The drawing under review shows one solid part. Ordinate dimensions are in mm from its lowest x, y, z. A direction names the side the tool comes from. Give positions to 0.01 mm unless a question says otherwise; leave off trailing zeros. Write each loop counter-clockwise with the first axis right and the second up, starting at its lowest first coordinate (ties: lowest second). Pieces come first, ordered by that corner, then holes. Notation, with made-up numbers: (53, -40) -> (59, -40) arc R19 cw to (59, -4) -> close; hole circle Ø11 at (59, 31.5). An arc over 180 degrees is marked (long way). Answer as a JSON object with one key per item and string values.
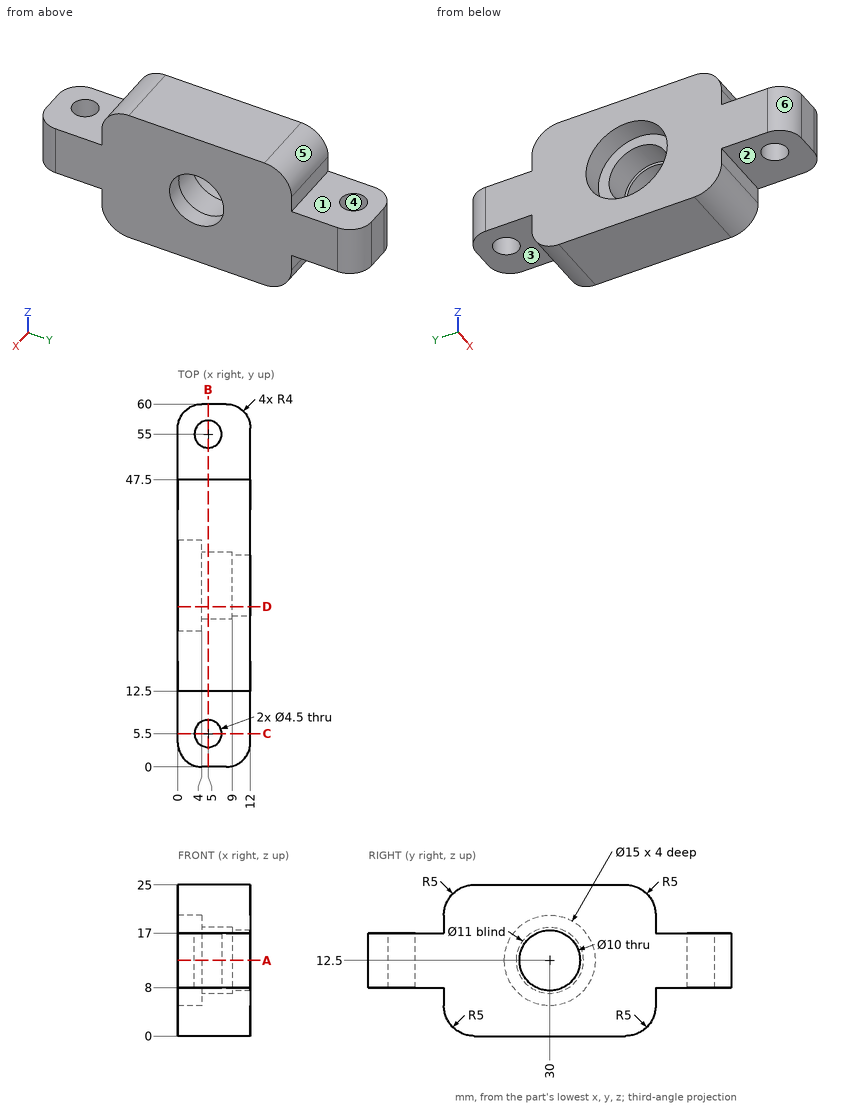
(1) For line 1 along Z through (x, y) = (6.75, 30); line 2 along Z through (x, y) = (9.75, 30); line 3 along Y through (x, z) = (7, 8.75), list the stretches that pass through material, from the lowest coordinate up.
Here are the results:
{"line 1": "z = 0 to 7, 18 to 25", "line 2": "z = 0 to 7.5, 17.5 to 25", "line 3": "y = 0 to 4.47, 6.53 to 25.98, 34.02 to 53.97, 56.03 to 60"}
(2) We need section A-A, the plane z = 12.5. State the section outline as (x, y) points, then the cut area to 3 significant figures.
Here are the results:
{"outline": "(0, 4) arc R4 ccw to (4, 0) -> (8, 0) arc R4 ccw to (12, 4) -> (12, 25) -> (9, 25) -> (9, 24.5) -> (4, 24.5) -> (4, 22.5) -> (0, 22.5) -> close; (0, 37.5) -> (4, 37.5) -> (4, 35.5) -> (9, 35.5) -> (9, 35) -> (12, 35) -> (12, 56) arc R4 ccw to (8, 60) -> (4, 60) arc R4 ccw to (0, 56) -> close; hole circle Ø4.5 at (5, 5.5); hole circle Ø4.5 at (5, 55)", "area": "529 mm²"}
(3) We need section D-D, the plane y = 26.5. State the section outline as (x, z) points, then the cut area to 3 significant figures.
Here are the results:
{"outline": "(0, 0) -> (12, 0) -> (12, 8.93) -> (9, 8.93) -> (9, 8.26) -> (4, 8.26) -> (4, 5.87) -> (0, 5.87) -> close; (0, 19.13) -> (4, 19.13) -> (4, 16.74) -> (9, 16.74) -> (9, 16.07) -> (12, 16.07) -> (12, 25) -> (0, 25) -> close", "area": "183 mm²"}
(4) We need section C-C, the plane y = 5.5. State the section outline as (x, z) points.
Here are the results:
{"outline": "(0, 8) -> (2.75, 8) -> (2.75, 17) -> (0, 17) -> close; (7.25, 8) -> (12, 8) -> (12, 17) -> (7.25, 17) -> close"}
(5) The part is to be moulded in two halves that separate along Y. For the marked faces 4, 5 and 6, say which applies: +Y half, -Y half, draft (parallel to the pull), parting line (faces both ways), or undercut.
Here are the results:
{"face 4": "undercut", "face 5": "+Y half", "face 6": "-Y half"}
(6) Clearance check with flat-ended pins moving along their axes: pin 1 (2.5 mm diameter, centred on x = 9, z = 18, fed in from -Y); pin 2 (3.5 mm diameter, centred on x = 6.5, z = 6, fed in from +Y); pin 3 (6 mm diameter, centred on x = 3, y = 52.5, fed in from -Z). State where each tip first meets the part, or that it passes through.
Here are the results:
{"pin 1": "stops at y = 0.01", "pin 2": "stops at y = 47.5", "pin 3": "stops at z = 8"}
(7) For the marked faces 1, 2 and 3, list the 3-axis set-ups (+Z, -Z, +X, -X, +Y, -Y) from which the entire face can be reached by the end or side of a thin tool; tool diameter is ignored.
Here are the results:
{"face 1": "+Z, +X, -X, +Y", "face 2": "-Z, +X, -X, -Y", "face 3": "-Z, +X, -X, +Y"}
(8) We need section B-B, the plane x = 5. State the section outline as (y, z) points.
Here are the results:
{"outline": "(0, 8) -> (3.25, 8) -> (3.25, 17) -> (0, 17) -> close; (7.75, 8) -> (12.5, 8) -> (12.5, 5) arc R5 ccw to (17.5, 0) -> (42.5, 0) arc R5 ccw to (47.5, 5) -> (47.5, 8) -> (52.75, 8) -> (52.75, 17) -> (47.5, 17) -> (47.5, 20) arc R5 ccw to (42.5, 25) -> (17.5, 25) arc R5 ccw to (12.5, 20) -> (12.5, 17) -> (7.75, 17) -> close; (57.25, 8) -> (60, 8) -> (60, 17) -> (57.25, 17) -> close; hole circle Ø11 at (30, 12.5)"}
